```python
from build123d import *

# Parameters (mm, degrees)
SKETCH036_R           = 2.25
PAD024_DEPTH          = 6
SKETCH038_W           = 20.5
SKETCH038_H           = 20.5
POCKET007_DEPTH       = 3
CYLINDER068_R         = 2.5
CYLINDER068_DEPTH     = 3
POLARPATTERN018_COUNT = 10
POLARPATTERN018_ANGLE = 140
POCKET009_DEPTH       = 2
POLARPATTERN019_COUNT = 4
POLARPATTERN019_ANGLE = 240


with BuildPart() as part:
    # Sketch036 → Pad024 (new body)
    with BuildSketch(Plane.YZ):
        with BuildLine():
            ThreePointArc((5.946308, -16.98945), (0, 18), (-5.946308, -16.98945))
            Line((-3.5, -10), (-5.946308, -16.98945))
            ThreePointArc((3.5, -10), (0, -6.5), (-3.5, -10))
            Line((5.946308, -16.98945), (3.5, -10))
        make_face()
        Circle(SKETCH036_R, mode=Mode.SUBTRACT)
    extrude(amount=PAD024_DEPTH)

    # Sketch038 (on Face6 of Pad024) → Pocket007 (cut)
    with BuildSketch(Plane(origin=(0, 0, 0), x_dir=(0, 1, 0), z_dir=(-1, 0, 0))):
        Rectangle(SKETCH038_W, SKETCH038_H)
    extrude(amount=-POCKET007_DEPTH, mode=Mode.SUBTRACT)

    # Cylinder068 → Cylinder068 (cut)
    with BuildSketch(Plane(origin=(0, 0, 18), x_dir=(0, 1, 0), z_dir=(1, 0, 0))):
        Circle(CYLINDER068_R)
    cylinder068 = extrude(amount=CYLINDER068_DEPTH, mode=Mode.SUBTRACT)

    # PolarPattern018: Cylinder068 ×10 about axis
    polarpattern018_axis = Axis((0, 0, 0), (-1, 0, 0))
    for i in range(1, POLARPATTERN018_COUNT):
        add(cylinder068.rotate(polarpattern018_axis, i * POLARPATTERN018_ANGLE / (POLARPATTERN018_COUNT - 1)), mode=Mode.SUBTRACT)

    # Sketch045 → Pocket009 (cut)
    with BuildSketch(Plane.YZ.offset(6)):
        with BuildLine():
            ThreePointArc((7.5, -12.990381), (12.990381, -7.5), (15, 0))
            Line((15, 0), (5, 0))
            ThreePointArc((2.5, -4.330127), (4.330127, -2.5), (5, 0))
            Line((2.5, -4.330127), (7.5, -12.990381))
        make_face()
    pocket009 = extrude(amount=-POCKET009_DEPTH, mode=Mode.SUBTRACT)

    # PolarPattern019: Pocket009 ×4 about axis
    polarpattern019_axis = Axis((6, 0, 0), (1, 0, 0))
    for i in range(1, POLARPATTERN019_COUNT):
        add(pocket009.rotate(polarpattern019_axis, i * POLARPATTERN019_ANGLE / (POLARPATTERN019_COUNT - 1)), mode=Mode.SUBTRACT)


with BuildPart() as part_1:
    # Body036 placement: moved
    add(part.part.moved(Location((-21, 0, 54))))


solid = part_1.part
```
Model file for the job. Use its own axes, mm. A direction names the side the tool comes from. Coordinates: 2 decimals unless noted, no trailing zeros. Loops run counter-clockwise (first coordinate to the right, second up) from the corner with the lowest first, then second, coordinate; pieces in that order, holes last. Notation, with made-up numbers: M 4.5,-24.75 L 21.5,-24.75 A22 cw 21.5,4.25 Z; hole C 3,-11.5 d10. An arc over 180 degrees is marked long. Use CSV: the item, a comma, the result in double quotes. Start each with the question number.
1. Band-saw the part on C-C, the plane z = 61. List the corners of the cut face in (x, y).
2. Tool access for faces 1 (the cylindrical face through (-16.52, -0.29, 56.23)), 2 (the cylindrical face through (-19.521, -0.412, 69.534)), 3 (the cylindrical face through (-19.521, 15.477, 53.141)), 4 (the cylindrical face through (-19.521, 11.246, 64.668)), 5 (the cylindrical face through (-16, -3, 58)): list every direction of +Z, -Z, +X, -X, +Y, -Y with a clear straight run to the whole face (end or side of a thin tool).
3. Band-saw the part on A-A, the plane x = -15.65. List the corners of the cut face in (y, z), then the cut area to 3 significant figures.
4. Band-saw the part on B-B, the plane y = 0. List the corners of the cut face in (x, z).
5. Two-plate mould, pull along Y, no slides. Class faces 6 (the flat face through (-15.986, 4.965, 45.4)), 7 (the cylindrical face through (-16, 3, 58)), 8 (the cylindrical face through (-19.52, 15.14, 57.32)): pulls with the +Y half, pulls with the -Y half, needs draft (parallel to the pull), parting line crosses it, or undercut.
6. Flat gauge pins, fed straight in: pin 1 (2.5 mm diameter, centred on x = -20, z = 51.5, fed in from -Y); pin 2 (3.5 mm diameter, centred on y = -11.5, z = 50.5, fed in from +X); pin 3 (10 mm diameter, centred on y = 8, z = 47.5, fed in from +X); pin 4 (2.5 mm diameter, centred on x = -19.5, y = 2, fed in from -Z). Where does each tip first touch, or does it go through?
7. Probe probe 1 along Z at (x, y) = (-15.7, 0); probe 2 along Y at (x, z) = (-17.35, 54); probe 3 along Z at (x, y) = (-15.55, -11). List the from-to ranges inside material, lowest first. Write a range as [from, to].
Entries:
1,outline,"M -21,-16.58 L -15,-16.58 L -15,-13.27 L -17,-13.27 L -17,-1.23 L -15,-1.23 L -15,1.23 L -17,1.23 L -17,13.27 L -15,13.27 L -15,16.58 L -18,16.58 L -18,13.85 L -21,13.85 L -21,10.25 L -18,10.25 L -18,-10.25 L -21,-10.25 Z"
2,face 1,"+X, -X"
2,face 2,"+Z, -X"
2,face 3,"-X, +Y"
2,face 4,"-X"
2,face 5,"+X"
3,outline,"M -5.95,37.01 L -3.5,44 A3.5 cw 3.5,44 L 5.95,37.01 A18 ccw long Z; hole M -15,54 A15 ccw -7.5,41.01 L -2.5,49.67 A5 cw -5,54 Z; hole M -14.1,59.13 L -4.7,55.71 A5 cw -0.87,58.92 L -2.6,68.77 A15 ccw Z; hole C 0,54 d4.5; hole M 0.87,58.92 A5 cw 4.7,55.71 L 14.1,59.13 A15 ccw 2.6,68.77 Z; hole M 2.5,49.67 L 7.5,41.01 A15 ccw 15,54 L 5,54 A5 cw Z"
3,area,"490 mm2"
4,outline,"M -21,64.25 L -18,64.25 L -18,56.25 L -15,56.25 L -15,72 L -18,72 L -18,69.5 L -21,69.5 Z; M -18,47.5 L -15,47.5 L -15,51.75 L -18,51.75 Z"
5,face 6,"undercut"
5,face 7,"undercut"
5,face 8,"pulls with the +Y half"
6,pin 1,"stops at y = -17.96"
6,pin 2,"stops at x = -17"
6,pin 3,"stops at x = -15"
6,pin 4,"stops at z = 64.25"
7,probe 1,"z = [47.5, 51.75], [56.25, 72]"
7,probe 2,"y = [-18, -2.25], [2.25, 18]"
7,probe 3,"z = [39.75, 43.8], [54, 58], [64.2, 68.25]"
